from build123d import *

# Parameters (mm, degrees)
BOSS_EXTRUDE1_DEPTH = 2.75
SKETCH3_R           = 1.5
CUT_EXTRUDE1_DEPTH  = 2.75
BOSS_EXTRUDE2_DEPTH = 2.75
SKETCH6_R           = 1.5
CUT_EXTRUDE2_DEPTH  = 2.75


with BuildPart() as part:
    # Sketch1 → Boss-Extrude1 (new body)
    with BuildSketch(Plane(origin=(0, 0, 0), x_dir=(1, 0, 0), z_dir=(0, 1, 0))):
        with BuildLine():
            Line((-7.5, 3.5), (7.5, 3.5))
            ThreePointArc((7.5, 3.5), (11, 0), (7.5, -3.5))
            Line((7.5, -3.5), (-7.5, -3.5))
            Line((-7.5, -3.5), (-7.5, 3.5))
        make_face()
    extrude(amount=BOSS_EXTRUDE1_DEPTH)

    # Sketch3 → Cut-Extrude1 (cut)
    with BuildSketch(Plane(origin=(0, 2.75, 0), x_dir=(1, 0, 0), z_dir=(0, 1, 0))):
        with Locations(Location((7.5, 0, 0), (0, 0, 270))):
            Circle(SKETCH3_R)
    extrude(amount=-CUT_EXTRUDE1_DEPTH, mode=Mode.SUBTRACT)

    # Sketch5 → Boss-Extrude2 (add)
    with BuildSketch(Plane.ZY.offset(7.5)):
        with BuildLine():
            Line((-3.5, 0), (3.5, 0))
            Line((3.5, 0), (3.5, 15))
            ThreePointArc((3.5, 15), (0, 18.5), (-3.5, 15))
            Line((-3.5, 15), (-3.5, 0))
        make_face()
    extrude(amount=-BOSS_EXTRUDE2_DEPTH)

    # Sketch6 → Cut-Extrude2 (cut)
    with BuildSketch(Plane(origin=(-4.75, 0, 0), x_dir=(0, 0, -1), z_dir=(1, 0, 0))):
        with Locations((0, 15)):
            Circle(SKETCH6_R)
    extrude(amount=-CUT_EXTRUDE2_DEPTH, mode=Mode.SUBTRACT)


solid = part.part
Can you work these out from the model? Positions are in its coordinate system, mm. A direction names the side the tool comes from. Give positions to 0.01 mm unless a question says otherwise; leave off trailing zeros. Order: outer loops, then holes, each group sorted by start corner. A loop starts at its lowest first (then second) coordinate and runs counter-clockwise, first axis right, second up. Notation, with made-up numbers: (-22, -14) - (-11, -14) arc R25 ccw to (-11, 17) - close; hole circle Ø3 at (45.25, -24). An arc over 180 degrees is marked (long way). Write each question's results on one line, items separated by ' | '.
1) Suppose I cut it at B-B, the plane y = 14.75. Write out the boundary of the cut face in (x, z).
Final values:
outline: (-7.5, -3.5) - (-4.75, -3.5) - (-4.75, -1.48) - (-7.5, -1.48) - close; (-7.5, 1.48) - (-4.75, 1.48) - (-4.75, 3.5) - (-7.5, 3.5) - close
2) Please list where these lines run through material, in increasing order: line 1 along X through (y, z) = (1.55, 0); line 2 along Y through (x, z) = (3.75, -2); line 3 along X through (y, z) = (10.5, -2.75). Write a range as [from, to].
Final values:
line 1: x = [-7.5, 6], [9, 11] | line 2: y = [0, 2.75] | line 3: x = [-7.5, -4.75]
3) Suppose I cut it at A-A, the plane z = 0. Write out the boundary of the cut face in (x, y), then the cut area to 3 significant figures.
Final values:
outline: (-7.5, 0) - (6, 0) - (6, 2.75) - (-4.75, 2.75) - (-4.75, 13.5) - (-7.5, 13.5) - close; (-7.5, 16.5) - (-4.75, 16.5) - (-4.75, 18.5) - (-7.5, 18.5) - close; (9, 0) - (11, 0) - (11, 2.75) - (9, 2.75) - close | area: 77.7 mm^2
4) Suppose I cut it at D-D, the plane y = 6. Write out the boundary of the cut face in (x, z), then the cut area to 4 significant figures.
Final values:
outline: (-7.5, -3.5) - (-4.75, -3.5) - (-4.75, 3.5) - (-7.5, 3.5) - close | area: 19.25 mm^2
5) Suppose I cut it at C-C, the plane x = -1.5. Write out the boundary of the cut face in (y, z), then the cut area to 4 significant figures.
Final values:
outline: (0, -3.5) - (2.75, -3.5) - (2.75, 3.5) - (0, 3.5) - close | area: 19.25 mm^2
6) If we mould it in two halves opening along Z, with no side actions, what happens to faces 1 (the face through (6, 1, 0)), 2 (the face through (3, 2.75, 0)), 3 (the face through (-6.11, 16.01, 1.11)), 4 (the face through (-6.1, 18.5, 0.1))? For each: pulls with the +Z half, pulls with the -Z half, needs draft (parallel to the pull), parting line crosses it, or undercut.
Final values:
face 1: undercut | face 2: needs draft | face 3: undercut | face 4: parting line crosses it
7) I'm going to push a flat-ended pin straight in: pin 1 Ø10 at (x, y) = (7, 3.5) entering from -Z. Where does the tip first touch, or does it pass through?
Final values:
pin 1: stops at z = -3.5
8) On a 3-axis mill with a long thin cutter (end or side, diameter ignored), from which of +Z, -Z, +X, -X, +Y, -Y can I reach the whole of each face in a straight line? I mean faces 5 (the face through (-3, 2, 3.5)), 6 (the face through (-4.75, 11, 0)). Say none if no direction works.
Final values:
face 5: +Z, +X, -X, +Y, -Y | face 6: +Z, -Z, +X, +Y
